Autodesk Inventor part; units mm, degrees
ref_plane "YZ Plane" through (0, 0, 0) normal (1, 0, 0) x (0, 1, 0)
ref_plane "XZ Plane" through (0, 0, 0) normal (0, 1, 0) x (-1, 0, 0)
ref_plane "XY Plane" through (0, 0, 0) normal (0, 0, 1) x (1, 0, 0)
sketch "Sketch1" plane through (0, 0, 0) normal (0, 1, 0) x (-1, 0, 0)
  line L0 (1.8436, -2.4426) -> (-23.5564, -2.4426)
  line L1 (-23.5564, -2.4426) -> (-23.5564, 22.9574)
  line L2 (-23.5564, 22.9574) -> (1.8436, 22.9574)
  line L3 (1.8436, 22.9574) -> (1.8436, -2.4426)
  line L4 (-20.3814, 0.7324) -> (-1.3314, 0.7324)
  line L5 (-1.3314, 0.7324) -> (-1.3314, 19.7824)
  line L6 (-1.3314, 19.7824) -> (-20.3814, 19.7824)
  line L7 (-20.3814, 19.7824) -> (-20.3814, 0.7324)
  point P0 (0, 0)
  dimension "d0" = 25.4
  dimension "d1" = 25.4
  dimension "d2" = 3.175
extrude "Extrusion1" add sketch "Sketch1" along normal blind 609.6
sketch "Sketch2" plane through (-1.8436, 0, -2.4426) normal (-1, 0, 0) x (0, 0, 1)
  line L0 (22.225, 0) -> (3.175, 0) construction
  line L1 (12.7, 0) -> (12.7, 12.7) construction
  line L2 (12.7, 12.7) -> (12.7, 38.1) construction
  line L3 (3.175, 609.6) -> (22.225, 609.6) construction
  line L4 (12.7, 609.6) -> (12.7, 596.9) construction
  line L5 (12.7, 596.9) -> (12.7, 571.5) construction
  circle A0 centre (12.7, 596.9) radius 2.5797
  circle A1 centre (12.7, 571.5) radius 2.5797
  circle A2 centre (12.7, 12.7) radius 2.5797
  circle A3 centre (12.7, 38.1) radius 2.5797
  point P0 (2.4426, 0)
  dimension "d5" = 12.7
  dimension "d6" = 25.4
  dimension "d7" = 12.7
  dimension "d8" = 25.4
  dimension "d9" = 5.1594
  dimension "d10" = 5.1594
  dimension "d11" = 5.1594
  dimension "d12" = 5.1594
extrude "Extrusion2" cut sketch "Sketch2" against normal blind 635
sketch "Sketch3" plane through (-1.8436, 0, -2.4426) normal (-1, 0, 0) x (0, 0, 1)
  circle A0 centre (12.7, 571.5) radius 2.5797 construction
  line L0 (12.7, 571.5) -> (12.7, 546.1) construction
  circle A1 centre (12.7, 546.1) radius 2.5797
  point P0 (2.4426, 0)
  dimension "d15" = 25.4
  dimension "d16" = 5.1594
extrude "Extrusion3" cut sketch "Sketch3" against normal blind 127
sketch "Sketch4" plane through (-1.8436, 0, 22.9574) normal (0, 0, 1) x (1, 0, 0)
  line L0 (0, 0) -> (25.4, 0) construction
  line L1 (12.7, 0) -> (12.7, 12.7) construction
  line L2 (12.7, 12.7) -> (12.7, 38.1) construction
  circle A0 centre (12.7, 12.7) radius 2.5797
  circle A1 centre (12.7, 38.1) radius 2.5797
  point P0 (1.8436, 0)
  dimension "d19" = 12.7
  dimension "d20" = 25.4
  dimension "d21" = 5.1594
  dimension "d22" = 5.1594
extrude "Extrusion4" cut sketch "Sketch4" against normal blind 127
properties part number "25in 1x1 Beam"
Geometry check sheet. Reference: the model listing, model coordinates, mm. A direction names the side the tool comes from. Give positions to 0.01 mm unless a question says otherwise; leave off trailing zeros. Write each loop counter-clockwise with the first axis right and the second up, starting at its lowest first coordinate (ties: lowest second). Pieces come first, ordered by that corner, then holes. Notation, with made-up numbers: M 15,18 L 52,18 A18 ccw 52,37 Z; hole C 72,-22.75 d8. An arc over 180 degrees is marked long. One line per question, with ' | ' between items.
1. Mould release check, pull along Z, two halves, no side actions. Record for faces 3 (the face through (20.381, 301, 10)), 4 (the face through (11, 301, 22.957)), 5 (the face through (11, 301, 19.782)), 6 (the face through (-1.844, 301, 10)): released by +Z, released by -Z, zero draft, split by the parting line, or undercut.
Ans:
face 3: undercut | face 4: released by +Z | face 5: undercut | face 6: zero draft
2. Scan lines: line 1 along X through (y, z) = (133.5, 12.75); line 2 along Z through (x, y) = (12.5, 162.5); line 3 along Z through (x, y) = (21.2, 571.5). Record each from-to range of solid material in increasing order. Write a range as from..to.
Ans:
line 1: -1.84..1.33, 20.38..23.56 | line 2: -2.44..0.73, 19.78..22.96 | line 3: -2.44..7.68, 12.84..22.96
3. Set-up check for faces 1 (the face through (23.556, 301, 10)), 2 (the face through (1.331, 301, 10)): record each of +Z, -Z, +X, -X, +Y, -Y from which the full face is reachable in a straight line by a thin tool's end or side.
Ans:
face 1: +Z, -Z, +X, +Y, -Y | face 2: +Y, -Y
4. Cross-section at A-A (y = 317). Enter the section's corners in (x, z), plus the area to 3 significant figures.
Ans:
outline: M -1.84,-2.44 L 23.56,-2.44 L 23.56,22.96 L -1.84,22.96 Z; hole M 1.33,0.73 L 20.38,0.73 L 20.38,19.78 L 1.33,19.78 Z | area: 282 mm2
5. Gauge pin test, flat end, axial feed: pin 1 (4.5 mm diameter, centred on y = 38.1, z = 10.26, fed in from +X). Record the tip position at first contact, or that the pin passes through.
Ans:
pin 1: through
